Check sheet for the drawn part. Datum: minimum x, y, z corner. Units: mm. A direction names the side the tool comes from. Coordinates: 2 decimals unless noted, no trailing zeros. Order: outer loops, then holes, each group sorted by start corner. A loop starts at its lowest first (then second) coordinate and runs counter-clockwise, first axis right, second up.
Q1. Cross-section at C-C, the plane z = 43. Record the boundary of the cut face in (x, y), and give its area (3 significant figures).
Q2. Draft check along X on the marked faces 1, 2 and 3. Enter one of: pulls with the +X half, pulls with the -X half, needs draft (parallel to the pull), parting line crosses it, or undercut.
Q3. Thickness scan on line 1 (X direction, y = 24.5, z = 62); line 2 (Y direction, x = 50, z = 66); line 3 (Y direction, x = 96.5, z = 39). Record the ranges inside material, lowest first.
Q4. Cross-section at A-A, the plane x = 50. Record the boundary of the cut face in (y, z).
Q5. Cross-section at B-B, the plane y = 25. Count the separate pieces of the cut face and the enclosed holes in it, and give its area (3 significant figures).
Q6. Set-up check for the marked faces 4 and 5: record each of +Z, -Z, +X, -X, +Y, -Y from which the full face is reachable in a straight line by a thin tool's end or side.
Q7. Depth check by flat-ended pin: P1, Ø1, axis at x = 72.5, y = 35.5, coming from the -Z side. Enter the tip coordinate at first touch or a pass-through.
Q8. Cross-section at D-D, the plane x = 25. Record the boundary of the cut face in (y, z), and give its area (3 significant figures).
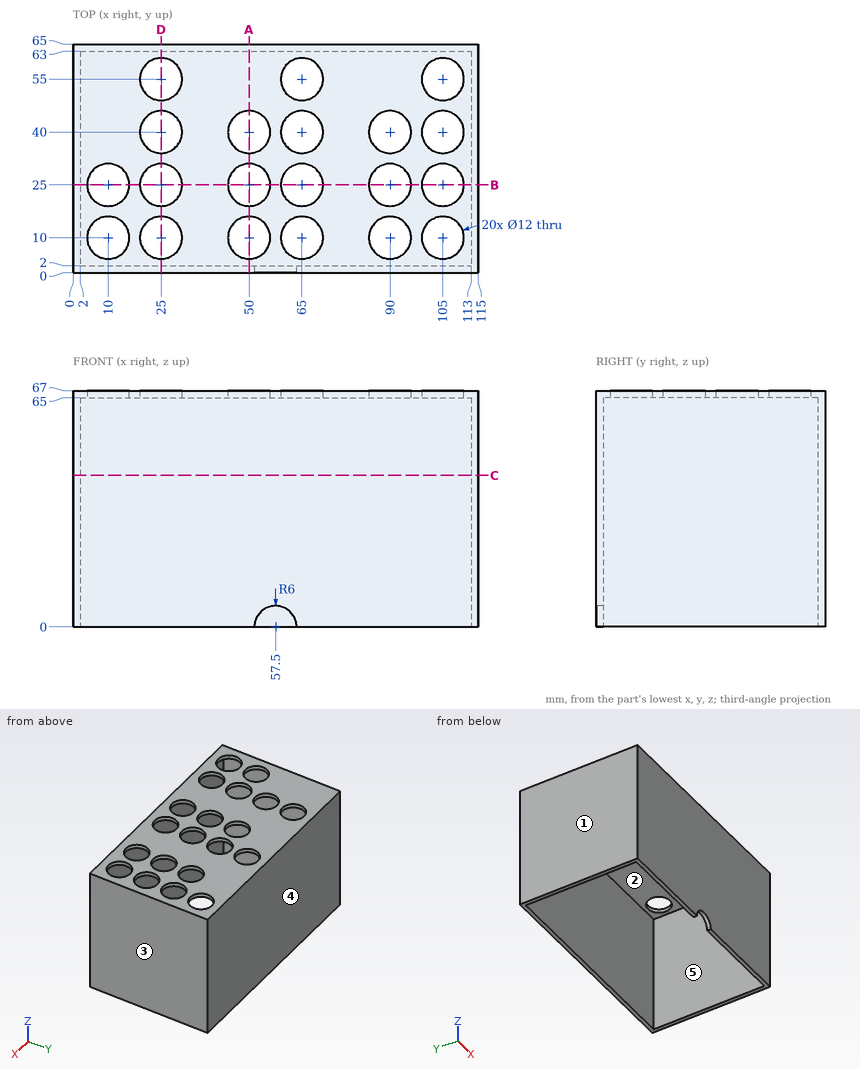
Check values:
1. outline: (0, 0) - (115, 0) - (115, 65) - (0, 65) - close; hole (2, 2) - (113, 2) - (113, 63) - (2, 63) - close
1. area: 704 mm2
2. face 1: pulls with the -X half
2. face 2: undercut
2. face 3: pulls with the +X half
3. line 1: x = 0 to 2, 113 to 115
3. line 2: y = 0 to 4, 16 to 19, 31 to 34, 46 to 65
3. line 3: y = 0 to 2, 63 to 65
4. outline: (0, 0) - (2, 0) - (2, 65) - (4, 65) - (4, 67) - (0, 67) - close; (16, 65) - (19, 65) - (19, 67) - (16, 67) - close; (31, 65) - (34, 65) - (34, 67) - (31, 67) - close; (46, 65) - (63, 65) - (63, 0) - (65, 0) - (65, 67) - (46, 67) - close
5. separate pieces: 7
5. enclosed holes: 0
5. area: 346 mm2
6. face 4: +Z, -Z, +X, -X, +Y
6. face 5: -Z
7. P1: stops at z = 65
8. outline: (0, 0) - (2, 0) - (2, 65) - (4, 65) - (4, 67) - (0, 67) - close; (16, 65) - (19, 65) - (19, 67) - (16, 67) - close; (31, 65) - (34, 65) - (34, 67) - (31, 67) - close; (46, 65) - (49, 65) - (49, 67) - (46, 67) - close; (61, 65) - (63, 65) - (63, 0) - (65, 0) - (65, 67) - (61, 67) - close
8. area: 294 mm2
